Check sheet for the modelled part. Datum: model origin and axes. Units: mm. Face numbers are marked on the shaded views. A direction names the side the tool comes from. Round coordinates to 2 decimals unless told otherwise and drop trailing zeros. Order: outer loops, then holes, each group sorted by start corner. A loop starts at its lowest first (then second) coordinate and runs counter-clockwise, first axis right, second up. Notation, with made-up numbers: (74, 53) -> (89, 53) arc R29 cw to (89, 90) -> close; hole circle Ø4 at (-19, 35.25). An arc over 180 degrees is marked (long way). Answer in a Markdown table with one row per item.
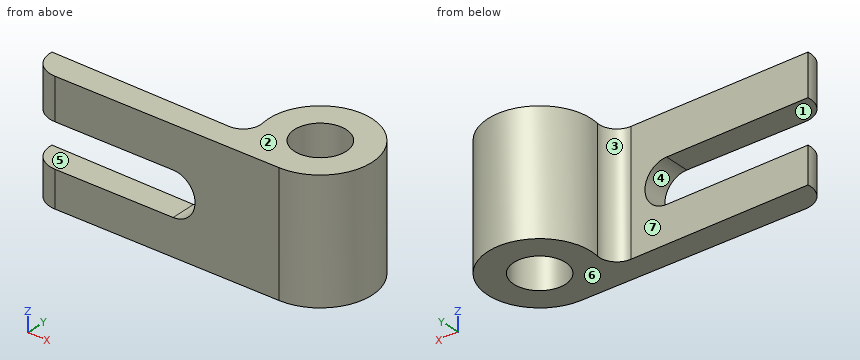
```python
from build123d import *

# Parameters (mm, degrees)
F1_DEPTH = 44.45
F2_R     = 9.525
F3_DEPTH = 50.8
F4_W     = 9.3673091604
F4_H     = 15.875
F5_DEPTH = 50.8


with BuildPart() as f1:
    # F0 (on Top) → F1 (new body)
    with BuildSketch(Plane.XY):
        with BuildLine():
            Line((-81.1569189035, -20.1813574524), (0.265105312, -19.0481552696))
            ThreePointArc((0.265105312, -19.0481552696), (12.2559693491, 14.584022604), (-18.8093233143, -3.0185851749))
            ThreePointArc((-18.8093233143, -3.0185851749), (-20.2463015318, -8.1438311785), (-25.0790977524, -10.3747802332))
            Line((-25.0790977524, -10.3747802332), (-35.6496162713, -10.3747802332))
            Line((-35.6496162713, -10.3747802332), (-78.4760718424, -10.3747802332))
            Line((-78.4760718424, -10.3747802332), (-81.139177084, -10.3747802332))
            Line((-81.139177084, -10.3747802332), (-90.1725590229, -10.3747802332))
            ThreePointArc((-90.1725590229, -10.3747802332), (-87.8582711897, -17.294684498), (-81.1569189035, -20.1813574524))
        make_face()
        with BuildLine():
            ThreePointArc((-81.2756354813, -10.3766794116), (-81.2074128903, -10.3752550508), (-81.139177084, -10.3747802332))
            Line((-81.139177084, -10.3747802332), (-81.2756354813, -10.3766794116))
        make_face(mode=Mode.SUBTRACT)
        with BuildLine():
            Line((-81.2756354813, -10.3766794116), (-81.139177084, -10.3747802332))
            ThreePointArc((-81.139177084, -10.3747802332), (-81.2074128903, -10.3752550508), (-81.2756354813, -10.3766794116))
        make_face()
    extrude(amount=F1_DEPTH)

    # F2 (on Top) → F3 (cut)
    with BuildSketch(Plane.XY):
        Circle(F2_R)
    extrude(amount=F3_DEPTH, mode=Mode.SUBTRACT)

    # F4 (on face) → F5 (cut)
    with BuildSketch(Plane(origin=(0, -10.3747802332, 0), x_dir=(-1, 0, 0), z_dir=(0, 1, 0))):
        with BuildLine():
            Line((38.230586797, 13.324032113), (77.2564191149, 13.324032113))
            Line((77.2564191149, 13.324032113), (77.2564191149, 29.199032113))
            Line((77.2564191149, 29.199032113), (38.230586797, 29.199032113))
            ThreePointArc((38.230586797, 29.199032113), (30.293086797, 21.261532113), (38.230586797, 13.324032113))
        make_face()
        with Locations((81.9400736951, 21.261532113)):
            Rectangle(F4_W, F4_H)
        Polygon((86.6237282753, 29.199032113), (86.6237282753, 13.324032113), (90.1725590229, 13.324032113), (98.23808074, 13.324032113), (98.23808074, 28.8764107972), (90.1725590229, 29.199032113), align=None)
    extrude(amount=-F5_DEPTH, mode=Mode.SUBTRACT)


solid = f1.part
```
(1) Depth check by flat-ended pin: pin 1 Ø3 at (x, z) = (-63.5, 5.5) entering from -Y; pin 2 Ø5 at (x, z) = (-3, 17) entering from -Y; pin 3 Ø1.5 at (y, z) = (-3.5, 34.5) entering from -X. Enter the tip coordinate at first touch or a pass-through.
Solutions:
| item | result |
|---|---|
| pin 1 | y = -19.96 |
| pin 2 | y = -19.13 |
| pin 3 | x = -18.85 |
(2) Draft check along Z on the marked faces 1, 2, 3 and 4. Enter one of: pulls with the +Z half, pulls with the -Z half, needs draft (parallel to the pull), parting line crosses it, or undercut.
Solutions:
| item | result |
|---|---|
| face 1 | undercut |
| face 2 | pulls with the +Z half |
| face 3 | needs draft |
| face 4 | undercut |
(3) Section check D-D on y = 13. Record the boundary of the cut face in (x, z), plus the area to 3 significant figures.
Solutions:
| item | result |
|---|---|
| outline | (-13.92, 0) -> (13.92, 0) -> (13.92, 44.45) -> (-13.92, 44.45) -> close |
| area | 1,240 mm^2 |
(4) Scan lines: probe 1 along Y at (x, z) = (0, 16) (3 decimals); probe 2 along X at (y, z) = (0, 28) (3 decimals); probe 3 along Z at (x, y) = (-60, -18). Record each from-to range of solid material in increasing order. Write a range as from..to.
Solutions:
| item | result |
|---|---|
| probe 1 | -19.052..-9.525, 9.525..19.05 |
| probe 2 | -19.05..-9.525, 9.525..19.05 |
| probe 3 | 0..13.32, 29.2..44.45 |
(5) Section check A-A on y = 0. Record the boundary of the cut face in (x, z) (3 decimals), plus the area to 3 significant figures.
Solutions:
| item | result |
|---|---|
| outline | (-19.05, 0) -> (-9.525, 0) -> (-9.525, 44.45) -> (-19.05, 44.45) -> close; (9.525, 0) -> (19.05, 0) -> (19.05, 44.45) -> (9.525, 44.45) -> close |
| area | 847 mm^2 |
(6) Section check C-C on z = 24. Record the boundary of the cut face in (x, y) (3 decimals), plus the area to 3 significant figures.
Solutions:
| item | result |
|---|---|
| outline | (-30.78, -19.48) -> (0.265, -19.048) arc R19.05 ccw (long way) to (-18.809, -3.019) arc R6.35 cw to (-25.079, -10.375) -> (-30.78, -10.375) -> close; hole circle Ø19.05 at (0, 0) |
| area | 1,050 mm^2 |
(7) Tool access check on the marked faces 5, 6 and 7. Record the directions out of +Z, -Z, +X, -X, +Y, -Y that give a thin tool (end or side, any length) a straight path to the whole face; none if there is none.
Solutions:
| item | result |
|---|---|
| face 5 | -X, +Y, -Y |
| face 6 | -Z, +X, -X, +Y, -Y |
| face 7 | +Z, -Z, -X, +Y |
(8) Section check B-B on x = -66. Record the boundary of the cut face in (y, z).
Solutions:
| item | result |
|---|---|
| outline | (-19.97, 0) -> (-10.37, 0) -> (-10.37, 13.32) -> (-19.97, 13.32) -> close; (-19.97, 29.2) -> (-10.37, 29.2) -> (-10.37, 44.45) -> (-19.97, 44.45) -> close |
